Geometry check sheet. Reference: the model listing, model coordinates, mm. A direction names the side the tool comes from. Give positions to 0.01 mm unless a question says otherwise; leave off trailing zeros. Write item = value, one per line. Start each with the question number.
(1) Access from +Z, -Z, +X, -X, +Y, -Y to the whole of each face (thin tool, end or side, straight path). Record for faces 4 (the cylindrical face through (-162.39, 271.97, 4.52)), 5 (the flat face through (-119, 6, 3)), 6 (the flat face through (-67, 273, 3)), 7 (the flat face through (-34, 276, 3)), 8 (the flat face through (-84, 140, 6)).
(2) Depth check by flat-ended pin: pin 1 Ø1 at (x, z) = (-102.5, 1) entering from -Y; pin 2 Ø2 at (x, z) = (-145.5, 2) entering from -Y; pin 3 Ø3 at (x, z) = (-79.5, 4) entering from +Y. Enter the tip coordinate at first touch or a pass-through.
(3) Thickness scan on L1, parallel to X at y = 273, z = 2.2; L2, parallel to Y at x = -101.5, z = 2 (3 decimals); L3, parallel to X at y = 143, z = 1.6. Record the ranges inside material, lowest first.
(4) Section check A-A, the plane z = 1.1. Give the number of separate pieces and of enclosed holes in the cut face, plus the area to 3 significant figures.
(5) Draft check along Y on faces 1 (the flat face through (-160.7, 141.7, 3)), 2 (the flat face through (-151, 36, 3)), 3 (the flat face through (-100, 3, 3)). Enter one of: pulls with the +Y half, pulls with the -Y half, needs draft (parallel to the pull), parting line crosses it, or undercut.
```python
from build123d import *

# Parameters (mm, degrees)
ESQUISSE1_W             = 165
ESQUISSE1_H             = 276
BOSS_EXTRU_1_DEPTH      = 6
ESQUISSE2_W             = 38
ESQUISSE2_H             = 6
ESQUISSE2_W_2           = 6
ESQUISSE2_H_2           = 32
ESQUISSE2_H_3           = 68
ESQUISSE2_W_3           = 40
EXTERIEUR_DEPTH         = 10
ESQUISSE3_R             = 11
ESQUISSE3_W             = 20
ESQUISSE3_H             = 6
ENL_V_MAT_EXTRU_2_DEPTH = 322.616230934
ESQUISSE4_R             = 1.5
ESQUISSE4_R_2           = 1.005
ENL_V_MAT_EXTRU_3_DEPTH = 322.616230934
ESQUISSE5_R             = 2.995
ESQUISSE5_R_2           = 3
ESQUISSE5_R_3           = 2
ENL_V_MAT_EXTRU_4_DEPTH = 3
ESQUISSE6_W             = 20
ESQUISSE6_H             = 110
ENL_V_MAT_EXTRU_5_DEPTH = 322.616230934


with BuildPart() as part:
    # Esquisse1 → Boss.-Extru.1 (new body)
    with BuildSketch(Plane.XY):
        with Locations((-82.5, 138)):
            Rectangle(ESQUISSE1_W, ESQUISSE1_H)
    extrude(amount=BOSS_EXTRU_1_DEPTH)

    # Esquisse2 → exterieur (cut)
    with BuildSketch(Plane.XY.offset(6)):
        with Locations((-86, 273)):
            Rectangle(ESQUISSE2_W, ESQUISSE2_H)
        with Locations((-162, 220)):
            Rectangle(ESQUISSE2_W_2, ESQUISSE2_H_2)
        with Locations((-162, 102)):
            Rectangle(ESQUISSE2_W_2, ESQUISSE2_H_3)
        Polygon((-137, 36), (-137, 6), (-100, 6), (-100, 0), (-165, 0), (-165, 36), align=None)
        with Locations((-40, 3)):
            Rectangle(ESQUISSE2_W_3, ESQUISSE2_H)
    extrude(amount=-EXTERIEUR_DEPTH, mode=Mode.SUBTRACT)

    # Esquisse3 → Enlèv. mat.-Extru.2 (cut, through all)
    with BuildSketch(Plane.XY.offset(6)):
        with Locations((-144, 178.92)):
            Circle(ESQUISSE3_R)
        with Locations((-135, 99)):
            Rectangle(ESQUISSE3_W, ESQUISSE3_H)
    extrude(amount=-ENL_V_MAT_EXTRU_2_DEPTH, mode=Mode.SUBTRACT)

    # Esquisse4 → Enlèv. mat.-Extru.3 (cut, through all)
    with BuildSketch(Plane.XY.offset(6)):
        with Locations((-32, 273)):
            Circle(ESQUISSE4_R)
        with Locations((-150, 273)):
            Circle(ESQUISSE4_R)
        with Locations((-162, 197)):
            Circle(ESQUISSE4_R)
        with Locations((-162, 170)):
            Circle(ESQUISSE4_R)
        with Locations((-162, 143)):
            Circle(ESQUISSE4_R)
        with Locations((-162, 61)):
            Circle(ESQUISSE4_R)
        with Locations((-162, 43)):
            Circle(ESQUISSE4_R)
        with Locations((-93, 3)):
            Circle(ESQUISSE4_R)
        with Locations((-67, 3)):
            Circle(ESQUISSE4_R)
        with Locations((-10, 3)):
            Circle(ESQUISSE4_R)
        with Locations((-152, 99)):
            Circle(ESQUISSE4_R)
        with Locations((-162, 243)):
            Circle(ESQUISSE4_R)
        with Locations((-101.5, 43)):
            Circle(ESQUISSE4_R_2)
        with Locations((-117.5, 43)):
            Circle(ESQUISSE4_R_2)
        with Locations((-101.5, 27)):
            Circle(ESQUISSE4_R_2)
        with Locations((-117.5, 27)):
            Circle(ESQUISSE4_R_2)
        with Locations((-162, 269)):
            Circle(ESQUISSE4_R)
    extrude(amount=-ENL_V_MAT_EXTRU_3_DEPTH, mode=Mode.SUBTRACT)

    # Esquisse5 → Enlèv. mat.-Extru.4 (cut)
    with BuildSketch(Plane.XY.offset(6)):
        with Locations((-150, 273)):
            Circle(ESQUISSE5_R)
        with Locations((-32, 273)):
            Circle(ESQUISSE5_R)
        with Locations((-162, 197)):
            Circle(ESQUISSE5_R)
        with Locations((-162, 170)):
            Circle(ESQUISSE5_R)
        with Locations((-162, 143)):
            Circle(ESQUISSE5_R)
        with Locations((-162, 61)):
            Circle(ESQUISSE5_R)
        with Locations((-162, 43)):
            Circle(ESQUISSE5_R)
        with Locations((-93, 3)):
            Circle(ESQUISSE5_R)
        with Locations((-67, 3)):
            Circle(ESQUISSE5_R)
        with Locations((-10, 3)):
            Circle(ESQUISSE5_R)
        with Locations((-152, 99)):
            Circle(ESQUISSE5_R_2)
        with Locations((-117.5, 43)):
            Circle(ESQUISSE5_R_3)
        with Locations((-101.5, 43)):
            Circle(ESQUISSE5_R_3)
        with Locations((-117.5, 27)):
            Circle(ESQUISSE5_R_3)
        with Locations((-101.5, 27)):
            Circle(ESQUISSE5_R_3)
        with Locations((-162, 269)):
            Circle(ESQUISSE5_R)
        with Locations((-162, 243)):
            Circle(ESQUISSE5_R)
    extrude(amount=-ENL_V_MAT_EXTRU_4_DEPTH, mode=Mode.SUBTRACT)

    # Esquisse6 → Enlèv. mat.-Extru.5 (cut, through all)
    with BuildSketch(Plane.XY.offset(6)):
        with Locations((-107, 126)):
            Rectangle(ESQUISSE6_W, ESQUISSE6_H)
    extrude(amount=-ENL_V_MAT_EXTRU_5_DEPTH, mode=Mode.SUBTRACT)


solid = part.part
```
Model answer:
q1.face_4 = +Z
q1.face_5 = +Z, -Z, -X, -Y
q1.face_6 = +Z, -Z, +Y
q1.face_7 = +Z, -Z, +X, -X, +Y
q1.face_8 = +Z, +X, -X, +Y, -Y
q2.pin_1 = 6
q2.pin_2 = 36
q2.pin_3 = 270
q3.L1 = -165 to -151.5, -148.5 to -105, -67 to -33.5, -30.5 to 0
q3.L2 = 6 to 25.995, 28.005 to 41.995, 44.005 to 71, 181 to 270
q3.L3 = -165 to -163.5, -160.5 to -117, -97 to 0
q4.separate_pieces = 1
q4.enclosed_holes = 20
q4.area = 40,400 mm²
q5.face_1 = undercut
q5.face_2 = pulls with the -Y half
q5.face_3 = needs draft
